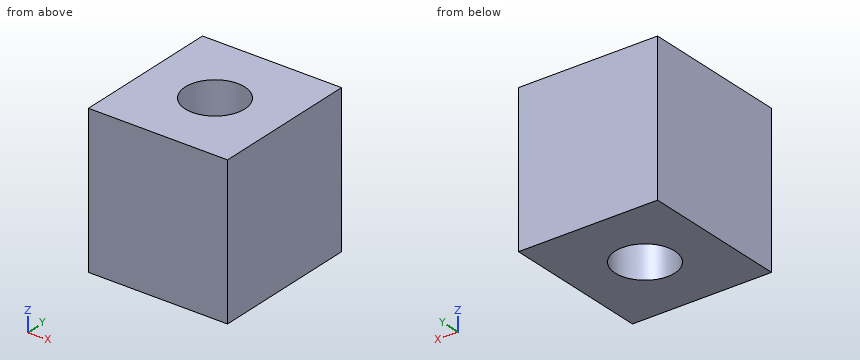
```python
from build123d import *

# Parameters (mm, degrees)
BOSS_EXTRUDE1_DEPTH = 30
SKETCH2_R           = 6
CUT_EXTRUDE1_DEPTH  = 45.676615807


with BuildPart() as part:
    # Sketch1 → Boss-Extrude1 (new body)
    with BuildSketch(Plane(origin=(0, 0, 0), x_dir=(1, 0, 0), z_dir=(0, 1, 0))):
        Polygon((-14, 0), (-14, -15), (14, -15), (14, 15), (-14, 15), align=None)
    extrude(amount=BOSS_EXTRUDE1_DEPTH)

    # Sketch2 → Cut-Extrude1 (cut, through all)
    with BuildSketch(Plane.XY.offset(15)):
        with Locations((0, 15)):
            Circle(SKETCH2_R)
    extrude(amount=-CUT_EXTRUDE1_DEPTH, mode=Mode.SUBTRACT)


solid = part.part
```
Source: CAD feature listing. Evaluate the final solid. Frame: model axes, mm. Coordinates: 2 decimals unless noted, no trailing zeros. Loops run counter-clockwise (first coordinate to the right, second up) from the corner with the lowest first, then second, coordinate; pieces in that order, holes last. Notation, with made-up numbers: M 7.5,-39 L 45.5,-39 A20 cw 45.5,0 Z; hole C 12,56 d9. An arc over 180 degrees is marked long. Use CSV: the item, a comma, the result in double quotes.
(1) Contact query for a flat-ended pin moving along its axis: pin 1 (3 mm diameter, centred on x = 1.5, z = -11, fed in from -Y). Output: stop coordinate, or through.
Answers follow:
pin 1,"y = 0"
(2) Cut plane C-C on z = -1.75. Return loops of the section in (x, y).
Answers follow:
outline,"M -14,0 L 14,0 L 14,30 L -14,30 Z; hole C 0,15 d12"
(3) Cut plane A-A on y = 15. Return loops of the section in (x, z), and give its area (3 significant figures).
Answers follow:
outline,"M -14,-15 L -6,-15 L -6,15 L -14,15 Z; M 6,-15 L 14,-15 L 14,15 L 6,15 Z"
area,"480 mm²"
(4) Cut plane B-B on x = 0. Return loops of the section in (y, z), and give its area (3 significant figures).
Answers follow:
outline,"M 0,-15 L 9,-15 L 9,15 L 0,15 Z; M 21,-15 L 30,-15 L 30,15 L 21,15 Z"
area,"540 mm²"
(5) Line query: line 1 (Y direction, x = 0, z = -8.25); line 2 (Y direction, x = -3, z = -5.5); line 3 (X direction, y = 9.5, z = 4.5). Output: solid intervals per line, ascending. Write a range as [from, to].
Answers follow:
line 1,"[0, 9], [21, 30]"
line 2,"[0, 9.8], [20.2, 30]"
line 3,"[-14, -2.4], [2.4, 14]"
